from build123d import *

# Parameters (mm, degrees)
SKETCH_1_R      = 3
SKETCH_1_R_2    = 1.5
EXTRUDE_1_DEPTH = 3
SKETCH_2_W      = 2
SKETCH_2_H      = 6
EXTRUDE_2_DEPTH = 15
SKETCH_3_W      = 3.5
SKETCH_3_H      = 26
EXTRUDE_3_DEPTH = 5
FILLET_1_R      = 3
FILLET_2_R      = 1.5


with BuildPart() as part:
    # 草图1 → 凸台-拉伸1 (new body)
    # profile 1 of 2: a face of its own
    with BuildSketch(Plane(origin=(0, 0, 0), x_dir=(1, 0, 0), z_dir=(0, 1, 0))):
        with BuildLine():
            Line((6, 3), (0, 3))
            ThreePointArc((0, 3), (2.121320344, 2.121320344), (3, 0))
            ThreePointArc((3, 0), (2.121320344, -2.121320344), (0, -3))
            Line((0, -3), (6, -3))
            Line((6, -3), (6, 3))
        make_face()
    # profile 2 of 2: a face of its own
    with BuildSketch(Plane(origin=(0, 0, 0), x_dir=(1, 0, 0), z_dir=(0, 1, 0))):
        Circle(SKETCH_1_R)
        with Locations(Location((0, 0, 0), (0, 0, 270))):
            Circle(SKETCH_1_R_2, mode=Mode.SUBTRACT)
    extrude(amount=EXTRUDE_1_DEPTH)

    # 草图2 → 凸台-拉伸2 (add)
    with BuildSketch(Plane(origin=(0, 0, 0), x_dir=(1, 0, 0), z_dir=(0, 1, 0))):
        with Locations((5, 0)):
            Rectangle(SKETCH_2_W, SKETCH_2_H)
    extrude(amount=EXTRUDE_2_DEPTH)

    # 草图3 → 凸台-拉伸3 (add)
    with BuildSketch(Plane(origin=(0, 15, 0), x_dir=(1, 0, 0), z_dir=(0, 1, 0))):
        Polygon((6, 3), (6, -63), (4, -63), (0.094051249, -63), (-1.5, -63), (-1.5, -33), (4, -33), (4, 3), align=None)
        with Locations((2.25, -48)):
            Rectangle(SKETCH_3_W, SKETCH_3_H, mode=Mode.SUBTRACT)
    extrude(amount=EXTRUDE_3_DEPTH)

    # 圆角1
    fillet_1_edges = [part.edges().sort_by_distance(p)[0] for p in [
        (5, 15, 3),
    ]]
    fillet(fillet_1_edges, radius=FILLET_1_R)

    # 圆角2
    fillet_2_edges = [part.edges().sort_by_distance(p)[0] for p in [
        (-1.5, 17.5, 33),
        (-1.5, 17.5, 63),
        (6, 17.5, 63),
        (4, 17.5, 35),
        (0.5, 17.5, 35),
        (0.5, 17.5, 61),
        (4, 17.5, 61),
    ]]
    fillet(fillet_2_edges, radius=FILLET_2_R)


solid = part.part
Here's how the part is built. I have some questions about the finished solid (model axes, mm). A direction names the side the tool comes from. Coordinates: 2 decimals unless noted, no trailing zeros. Order: outer loops, then holes, each group sorted by start corner. A loop starts at its lowest first (then second) coordinate and runs counter-clockwise, first axis right, second up. Notation, with made-up numbers: (49, -14.75) -> (87, -14.75) arc R26 ccw to (87, 11.25) -> close; hole circle Ø6 at (44.25, -30.75). An arc over 180 degrees is marked (long way). Answer in a Markdown table with one row per item.
(1) Please list where these lines run through material, in increasing order: probe 1 along X at (y, z) = (18, 49); probe 2 along X at (y, z) = (1.75, 0); probe 3 along Z at (x, y) = (4.75, 7).
Answer key:
| item | result |
|---|---|
| probe 1 | -1.5 to 0.5, 4 to 6 |
| probe 2 | -3 to -1.5, 1.5 to 6 |
| probe 3 | -3 to 3 |
(2) I want a section at C-C on z = 58. List the corners of the cut face in (x, y) for me, then the cut area to 3 significant figures.
Answer key:
| item | result |
|---|---|
| outline | (-1.5, 15) -> (0.5, 15) -> (0.5, 20) -> (-1.5, 20) -> close; (4, 15) -> (6, 15) -> (6, 20) -> (4, 20) -> close |
| area | 20.0 mm^2 |
(3) On a 3-axis mill with a long thin cutter (end or side, diameter ignored), from which of +Z, -Z, +X, -X, +Y, -Y can I reach the whole of each face in a straight line? I mean faces 4 (the face through (3.55, 17.54, 35.43)), 5 (the face through (2, 17, 33)), 6 (the face through (4, 15.2, 11.3)), 7 (the face through (4.3, 4.6, 3)). Say none if no direction works.
Answer key:
| item | result |
|---|---|
| face 4 | +Y, -Y |
| face 5 | -Z, -X, +Y, -Y |
| face 6 | -Z, -X, +Y |
| face 7 | +Z, +X, -X, -Y |
(4) I want a section at D-D on z = 27.5. List the corners of the cut face in (x, y) for me.
Answer key:
| item | result |
|---|---|
| outline | (4, 15) -> (6, 15) -> (6, 20) -> (4, 20) -> close |
(5) Will these pins go through, and if not, where does the flat tip stop? pin 1 Ø1.5 at (y, z) = (16.5, 49.5) entering from -X; pin 2 Ø5 at (x, y) = (3.5, 7.5) entering from +Z; pin 3 Ø2 at (x, y) = (2.5, 17.5) entering from -Z; pin 4 Ø1 at (y, z) = (13.5, 40) entering from -X.
Answer key:
| item | result |
|---|---|
| pin 1 | x = -1.5 |
| pin 2 | z = 3 |
| pin 3 | z = 33 |
| pin 4 | through |
(6) Thinking about a two-plate mould opening in X: for faces 1 (the face through (0.5, 17, 48)), 2 (the face through (-1.5, 17, 48)), 3 (the face through (2, 0, 0)), which applies, +X half, -X half, draft (parallel to the pull), parting line (faces both ways), or undercut?
Answer key:
| item | result |
|---|---|
| face 1 | undercut |
| face 2 | -X half |
| face 3 | draft |
(7) I want a section at A-A on z = 0. List the corners of the cut face in (x, y) for me, then the cut area to 3 significant figures.
Answer key:
| item | result |
|---|---|
| outline | (-3, 0) -> (-1.5, 0) -> (-1.5, 3) -> (-3, 3) -> close; (1.5, 0) -> (6, 0) -> (6, 20) -> (4, 20) -> (4, 3) -> (1.5, 3) -> close |
| area | 52.0 mm^2 |
(8) I want a section at B-B on y = 16.25. List the corners of the cut face in (x, z) for me, then the cut area to 3 significant figures.
Answer key:
| item | result |
|---|---|
| outline | (-1.5, 34.5) arc R1.5 ccw to (0, 33) -> (4, 33) -> (4, -3) -> (6, -3) -> (6, 61.5) arc R1.5 ccw to (4.5, 63) -> (0, 63) arc R1.5 ccw to (-1.5, 61.5) -> close; hole (0.5, 36.5) arc R1.5 ccw to (2, 35) -> (2.5, 35) arc R1.5 ccw to (4, 36.5) -> (4, 59.5) arc R1.5 ccw to (2.5, 61) -> (2, 61) arc R1.5 ccw to (0.5, 59.5) -> close |
| area | 206 mm^2 |
